Could you check a few things on this model? Use its own coordinates, in mm. A direction names the side the tool comes from. Give positions to 0.01 mm unless a question says otherwise; leave off trailing zeros. Loops run counter-clockwise (first coordinate to the right, second up) from the corner with the lowest first, then second, coordinate; pieces in that order, holes last. Notation, with made-up numbers: M 81.25,-27.75 L 120.25,-27.75 A18 cw 120.25,-9.75 Z; hole C 40.5,-35.5 d11. An arc over 180 degrees is marked long. Use a Markdown table: item, result. Add a question column.
1) Suppose I cut it at B-B on y = 0. List the corners of the cut face in (x, z) for me, and give its area (3 significant figures).
2) Suppose I cut it at D-D on x = 11. List the corners of the cut face in (y, z) for me.
3) Which directions (+Z, -Z, +X, -X, +Y, -Y) give clear straight access to the entire face, cutting with the end or side of a thin tool? Please do faces 1 (the cylindrical face through (-6.01, 7.76, 4.03)), 2 (the flat face through (-8, 8, 2)), 3 (the flat face through (9, -19, 4)).
4) We'd pull the mould along Y, two halves only. Please class faces 4 (the flat face through (0, 0, 6)), 5 (the flat face through (-8, -6, 2)), 6 (the cylindrical face through (4.336, -19.524, 4.986)): +Y half, -Y half, draft (parallel to the pull), parting line (faces both ways), or undercut.
5) If I drill on line 1 along Y through (x, z) = (8.5, 0.65); line 2 along Y through (x, z) = (-7, 1.55), over which ranges is the centre line in solid material (lowest first)? Write a range as [from, to].
6) Suppose I cut it at C-C on x = -7. List the corners of the cut face in (y, z) for me (3 decimals).
7) Will these pins go through, and if not, where does the flat tip stop? pin 1 Ø4 at (x, y) = (17, -23) entering from -Z; pin 2 Ø2 at (x, z) = (-3.5, 4) entering from +Y; pin 3 Ø1.2 at (x, y) = (6.5, -8) entering from -Z.
8) Suppose I cut it at A-A on z = 0.9. List the corners of the cut face in (x, y) for me.
Autodesk Fusion 360 part; units mm, degrees
sketch "Base" plane through (0, 0, 0) normal (0, 0, 1) x (1, 0, 0)
  circle A0 centre (0, 0) radius 45
  dimension "d1" = 90
extrude "Extrude1" add sketch "Base" along normal blind 4
sketch "Stand" plane through (0, 0, 4) normal (0, 0, 1) x (-1, 0, 0)
  circle A0 centre (0, 0) radius 45
  circle A1 centre (0, 0) radius 20
  dimension "d4" = 40
extrude "Extrude2" add sketch "Stand" along normal blind 2 contours A1
sketch "Holes" plane through (0, 0, 6) normal (0, 0, 1) x (-1, 0, 0)
  circle A0 centre (0, 0) radius 20
  circle A1 centre (7, -7) radius 1.25
  circle A2 centre (-7, -7) radius 1.25
  line L0 (20, 0) -> (20, -20)
  line L1 (20, -20) -> (0, -20)
  line L2 (-20, 0) -> (-20, 20)
  line L3 (-20, 20) -> (0, 20)
  line L4 (20, -20) -> (-20, -20)
  line L5 (-20, -20) -> (-20, 20)
  line L6 (-20, 20) -> (20, 20)
  line L7 (20, 20) -> (20, -20)
  circle A3 centre (7, 7) radius 1.25
  circle A4 centre (-7, 7) radius 1.25
  dimension "d7" = 2.5
  dimension "d8" = 2.5
  dimension "d10" = 13
  dimension "d11" = 13
  dimension "d12" = 13
  dimension "d13" = 13
  dimension "d14" = 2.5
  dimension "d15" = 2.5
  dimension "d16" = 13
  dimension "d17" = 13
  dimension "d18" = 13
  dimension "d19" = 13
extrude "Extrude3" cut sketch "Holes" against normal blind 6 contours A1 | A2 | A3 | A4
sketch "Fillets" plane through (0, 0, 0) normal (0, 0, -1) x (1, 0, 0)
  circle A0 centre (7, -7) radius 1.25
  circle A1 centre (-7, 7) radius 1.25
  circle A2 centre (-7, -7) radius 1.25
  circle A3 centre (7, 7) radius 1.25
  circle A4 centre (0, 0) radius 45
  circle A5 centre (-7, 7) radius 2
  circle A6 centre (7, 7) radius 2
  circle A7 centre (-7, -7) radius 2
  circle A8 centre (7, -7) radius 2
  dimension "d27" = 4
  dimension "d28" = 4
  dimension "d29" = 4
  dimension "d30" = 4
extrude "Extrude5" cut sketch "Fillets" against normal blind 2 contours A5 | A6 | A7 | A8
Answer block:
| question | item | result |
|---|---|---|
| 1 | outline | M -45,0 L 45,0 L 45,4 L 20,4 L 20,6 L -20,6 L -20,4 L -45,4 Z |
| 1 | area | 440 mm^2 |
| 2 | outline | M -43.63,0 L 43.63,0 L 43.63,4 L 16.7,4 L 16.7,6 L -16.7,6 L -16.7,4 L -43.63,4 Z |
| 3 | face 1 | +Z, -Z |
| 3 | face 2 | -Z |
| 3 | face 3 | +Z |
| 4 | face 4 | draft |
| 4 | face 5 | undercut |
| 4 | face 6 | parting line |
| 5 | line 1 | y = [-44.19, -8.32], [-5.68, 5.68], [8.32, 44.19] |
| 5 | line 2 | y = [-44.45, -9], [-5, 5], [9, 44.45] |
| 6 | outline | M -44.452,0 L -9,0 L -9,2 L -8.25,2 L -8.25,6 L -18.735,6 L -18.735,4 L -44.452,4 Z; M -5.75,2 L -5,2 L -5,0 L 5,0 L 5,2 L 5.75,2 L 5.75,6 L -5.75,6 Z; M 8.25,2 L 9,2 L 9,0 L 44.452,0 L 44.452,4 L 18.735,4 L 18.735,6 L 8.25,6 Z |
| 7 | pin 1 | stops at z = 0 |
| 7 | pin 2 | stops at y = 44.93 |
| 7 | pin 3 | stops at z = 2 |
| 8 | outline | C 0,0 d90; hole C -7,-7 d4; hole C -7,7 d4; hole C 7,-7 d4; hole C 7,7 d4 |
